```python
from build123d import *

# Parameters (mm, degrees)
SKETCH1_W               = 27
SKETCH1_H               = 10.1
SKETCH1_W_2             = 24
SKETCH1_H_2             = 7.1
SKETCH1_R               = 2.5
SKETCH1_R_2             = 1.55
BOSS_EXTRUDE2_DEPTH     = 10
CUT_EXTRUDE2_START      = 10
SKETCH1_5_R             = 2.5
SKETCH1_5_R_2           = 1.55
CUT_EXTRUDE2_DEPTH      = 2.7
FILLET1_R               = 3
CUT_EXTRUDE3_START      = 7.8
SKETCH1_6_W             = 24
SKETCH1_6_H             = 7.1
SKETCH1_6_R             = 2.5
SKETCH1_6_R_2           = 1.55
CUT_EXTRUDE3_DEPTH      = 6.5
SKETCH2_R               = 1.475
CUT_EXTRUDE4_DEPTH      = 25
CUT_EXTRUDE5_DEPTH      = 30.23187487
CUT_EXTRUDE5_DEPTH_BACK = 30.23187487
SKETCH2_3_R             = 1.475
SKETCH3_R               = 0.9
CUT_EXTRUDE6_DEPTH      = 18.54287621


with BuildPart() as part:
    # Sketch1 → Boss-Extrude2 (new body)
    # profile 1 of 5: a face of its own
    with BuildSketch(Plane(origin=(0, 0, 0), x_dir=(1, 0, 0), z_dir=(0, 1, 0))):
        Rectangle(SKETCH1_W, SKETCH1_H)
        Rectangle(SKETCH1_W_2, SKETCH1_H_2, mode=Mode.SUBTRACT)
    # profile 2 of 5: a face of its own
    with BuildSketch(Plane(origin=(0, 0, 0), x_dir=(1, 0, 0), z_dir=(0, 1, 0))):
        Rectangle(SKETCH1_W_2, SKETCH1_H_2)
        with Locations((6, 0)):
            Circle(SKETCH1_R, mode=Mode.SUBTRACT)
        Circle(SKETCH1_R_2, mode=Mode.SUBTRACT)
        with Locations((-6, 0)):
            Circle(SKETCH1_R, mode=Mode.SUBTRACT)
    # profile 3 of 5: a face of its own
    with BuildSketch(Plane(origin=(0, 0, 0), x_dir=(1, 0, 0), z_dir=(0, 1, 0))):
        with Locations((-6, 0)):
            Circle(SKETCH1_R)
    # profile 4 of 5: a face of its own
    with BuildSketch(Plane(origin=(0, 0, 0), x_dir=(1, 0, 0), z_dir=(0, 1, 0))):
        Circle(SKETCH1_R_2)
    # profile 5 of 5: a face of its own
    with BuildSketch(Plane(origin=(0, 0, 0), x_dir=(1, 0, 0), z_dir=(0, 1, 0))):
        with Locations((6, 0)):
            Circle(SKETCH1_R)
    extrude(amount=BOSS_EXTRUDE2_DEPTH)

    # Sketch1<5> → Cut-Extrude2 (cut)
    with BuildSketch(Plane(origin=(0, 0, 0), x_dir=(1, 0, 0), z_dir=(0, 1, 0)).offset(CUT_EXTRUDE2_START)):
        with Locations(Location((6, 0, 0), (0, 0, 270))):
            Circle(SKETCH1_5_R)
        with Locations(Location((0, 0, 0), (0, 0, 270))):
            Circle(SKETCH1_5_R_2)
        with Locations(Location((-6, 0, 0), (0, 0, 270))):
            Circle(SKETCH1_5_R)
    extrude(amount=-CUT_EXTRUDE2_DEPTH, mode=Mode.SUBTRACT)

    # Fillet1
    # the kernel refuses this fillet: 3 mm, written as the material it takes off along each edge
    with BuildSketch(Plane(origin=(21, 10, 5.05), x_dir=(0, 0, -1), z_dir=(-1, 0, 0)), Plane(origin=(-21, 0, -5.05), x_dir=(0, 1, 0), z_dir=(1, 0, 0))) as fillet1_piece_1:
        with BuildLine():
            CenterArc((FILLET1_R, FILLET1_R), FILLET1_R, 180, 90)
            Line((0, FILLET1_R), (0, 0))
            Line((0, 0), (FILLET1_R, 0))
        make_face()
    extrude(amount=42, mode=Mode.SUBTRACT)
    with BuildSketch(Plane(origin=(-21, 10, -5.05), x_dir=(0, -1, 0), z_dir=(1, 0, 0)), Plane(origin=(21, 0, 5.05), x_dir=(0, 0, -1), z_dir=(-1, 0, 0))) as fillet1_piece_2:
        with BuildLine():
            CenterArc((FILLET1_R, -FILLET1_R), FILLET1_R, 90, 90)
            Line((0, -FILLET1_R), (0, 0))
            Line((0, 0), (FILLET1_R, 0))
        make_face()
    extrude(amount=42, mode=Mode.SUBTRACT)

    # Sketch1<6> → Cut-Extrude3 (cut)
    with BuildSketch(Plane(origin=(0, 0, 0), x_dir=(1, 0, 0), z_dir=(0, 1, 0)).offset(CUT_EXTRUDE3_START)):
        Rectangle(SKETCH1_6_W, SKETCH1_6_H)
        with Locations(Location((6, 0, 0), (0, 0, 270))):
            Circle(SKETCH1_6_R, mode=Mode.SUBTRACT)
        with Locations(Location((0, 0, 0), (0, 0, 270))):
            Circle(SKETCH1_6_R_2, mode=Mode.SUBTRACT)
        with Locations(Location((-6, 0, 0), (0, 0, 270))):
            Circle(SKETCH1_6_R, mode=Mode.SUBTRACT)
    extrude(amount=-CUT_EXTRUDE3_DEPTH, mode=Mode.SUBTRACT)

    # Sketch2 → Cut-Extrude4 (cut)
    # profile 1 of 2: a face of its own
    with BuildSketch(Plane(origin=(13.5, 0, 0), x_dir=(0, 0, -1), z_dir=(1, 0, 0))):
        with BuildLine():
            Line((2.05, 8.5), (-2.05, 8.5))
            ThreePointArc((-2.05, 8.5), (-3.110660172, 8.060660172), (-3.55, 7))
            Line((-3.55, 7), (-3.55, 3))
            ThreePointArc((-3.55, 3), (-3.110660172, 1.939339828), (-2.05, 1.5))
            Line((-2.05, 1.5), (2.05, 1.5))
            ThreePointArc((2.05, 1.5), (3.110660172, 1.939339828), (3.55, 3))
            Line((3.55, 3), (3.55, 7))
            ThreePointArc((3.55, 7), (3.110660172, 8.060660172), (2.05, 8.5))
        make_face()
        with Locations((0, 5)):
            Circle(SKETCH2_R, mode=Mode.SUBTRACT)
    # profile 2 of 2: a face of its own
    with BuildSketch(Plane(origin=(13.5, 0, 0), x_dir=(0, 0, -1), z_dir=(1, 0, 0))):
        with Locations((0, 5)):
            Circle(SKETCH2_R)
    extrude(amount=-CUT_EXTRUDE4_DEPTH, mode=Mode.SUBTRACT)

    # Sketch2<3> → Cut-Extrude5 (cut, two sides: drawn at the far end of the back side and taken through both)
    with BuildSketch(Plane(origin=(13.5, 0, 0), x_dir=(0, 0, -1), z_dir=(1, 0, 0)).offset(-CUT_EXTRUDE5_DEPTH_BACK)):
        with Locations((0, 5)):
            Circle(SKETCH2_3_R)
    extrude(amount=CUT_EXTRUDE5_DEPTH + CUT_EXTRUDE5_DEPTH_BACK, mode=Mode.SUBTRACT)

    # Sketch3 → Cut-Extrude6 (cut, through all)
    with BuildSketch(Plane(origin=(0, 0, 0), x_dir=(1, 0, 0), z_dir=(0, -0.7071067811865475, 0.7071067811865477))):
        with Locations(Location((0, 3.570889245, 0), (0, 0, 90))):
            Circle(SKETCH3_R)
    extrude(amount=CUT_EXTRUDE6_DEPTH, mode=Mode.SUBTRACT)


solid = part.part
```
Verification items for the finished model (mm, model axes). A direction names the side the tool comes from. Coordinates: 2 decimals unless noted, no trailing zeros. Write each loop counter-clockwise with the first axis right and the second up, starting at its lowest first coordinate (ties: lowest second). Pieces come first, ordered by that corner, then holes. Notation, with made-up numbers: M -14.75,-32 L -0.75,-32 A15 ccw -0.75,-8 Z; hole C 8,-9 d1. An arc over 180 degrees is marked long. One line per item, written item: value.
Item 1: Section check A-A, the plane y = 5. Record the boundary of the cut face in (x, z) (3 decimals), plus the area to 3 significant figures.
Check sheet entries:
outline: M -13.5,-5.05 L 13.5,-5.05 L 13.5,-3.55 L -12,-3.55 L -12,-1.475 L -13.5,-1.475 Z; M -13.5,1.475 L -12,1.475 L -12,3.55 L 13.5,3.55 L 13.5,5.05 L -13.5,5.05 Z
area: 87.2 mm^2
Item 2: Mould release check, pull along Y, two halves, no side actions. Record for faces 6 (the cylindrical face through (-0.19, 9.1, -4.19)), 7 (the flat face through (1, 5, -3.55)), 8 (the cylindrical face through (12.76, 1.95, 3.12)), 9 (the cylindrical face through (0.466, 9.26, 1.478)): pulls with the +Y half, pulls with the -Y half, needs draft (parallel to the pull), parting line crosses it, or undercut.
Check sheet entries:
face 6: pulls with the +Y half
face 7: undercut
face 8: undercut
face 9: needs draft
Item 3: Section check C-C, the plane z = 0. State how many separate pieces and enclosed holes the cut face has, plus the area to 3 significant figures.
Check sheet entries:
separate pieces: 5
enclosed holes: 0
area: 65.6 mm^2
Item 4: Gauge pin test, flat ends, axial feed: pin 1 Ø1.9 at (x, z) = (0, 0) entering from +Y; pin 2 Ø0.6 at (y, z) = (8, 1.5) entering from +X. Record the tip position at first contact, or that the pin passes through.
Check sheet entries:
pin 1: stops at y = 1.5
pin 2: stops at x = -11.5
Item 5: Scan lines: line 1 along X through (y, z) = (8.8, 0); line 2 along Z through (x, y) = (-3.5, 5); line 3 along Z through (x, y) = (-12.9, 5) (3 decimals). Record each from-to range of solid material in increasing order.
Check sheet entries:
line 1: x = -13.5 to -8.5, -3.5 to -1.55, 1.55 to 3.5, 8.5 to 13.5
line 2: z = -5.05 to -3.55, 3.55 to 5.05
line 3: z = -5.05 to -1.475, 1.475 to 5.05
Item 6: Section check B-B, the plane x = 0. Record the boundary of the cut face in (y, z).
Check sheet entries:
outline: M 0,-2.05 A3 ccw 3,-5.05 L 7,-5.05 A3 ccw 10,-2.05 L 10,-1.55 L 8.5,-1.55 L 8.5,-2.05 A1.5 cw 7.8,-3.32 L 7.8,-3.55 L 1.3,-3.55 L 1.3,-1.55 L 1.5,-1.55 L 1.5,1.55 L 1.3,1.55 L 1.3,2.48 L 0.34,3.44 A3 ccw 0,2.05 Z; M 1.61,4.71 L 2.77,3.55 L 7.8,3.55 L 7.8,3.32 A1.5 cw 8.5,2.05 L 8.5,1.55 L 10,1.55 L 10,2.05 A3 ccw 7,5.05 L 3,5.05 A3 ccw Z
Item 7: Section check D-D, the plane x = 6. Record the boundary of the cut face in (y, z).
Check sheet entries:
outline: M 0,-2.05 A3 ccw 3,-5.05 L 7,-5.05 A3 ccw 9.97,-2.5 L 8.43,-2.5 A1.5 cw 7.8,-3.32 L 7.8,-3.55 L 1.3,-3.55 L 1.3,-2.5 L 1.57,-2.5 A1.5 cw 1.5,-2.05 L 1.5,2.05 A1.5 cw 1.57,2.5 L 1.3,2.5 L 1.3,3.55 L 7.8,3.55 L 7.8,3.32 A1.5 cw 8.43,2.5 L 9.97,2.5 A3 ccw 7,5.05 L 3,5.05 A3 ccw 0,2.05 Z
Item 8: Access from +Z, -Z, +X, -X, +Y, -Y to the whole of each face (thin tool, end or side, straight path). Record for faces 1 (the cylindrical face through (12.76, 1.93, -3.1)), 2 (the cylindrical face through (-3.89, 9.23, 1.34)), 3 (the flat face through (13.5, 9, 0)), 4 (the flat face through (0, 1.3, -2)), 5 (the flat face through (0, 1.5, 0)).
Check sheet entries:
face 1: +X
face 2: +Y
face 3: +Z, -Z, +X, +Y, -Y
face 4: none
face 5: +X, +Y
